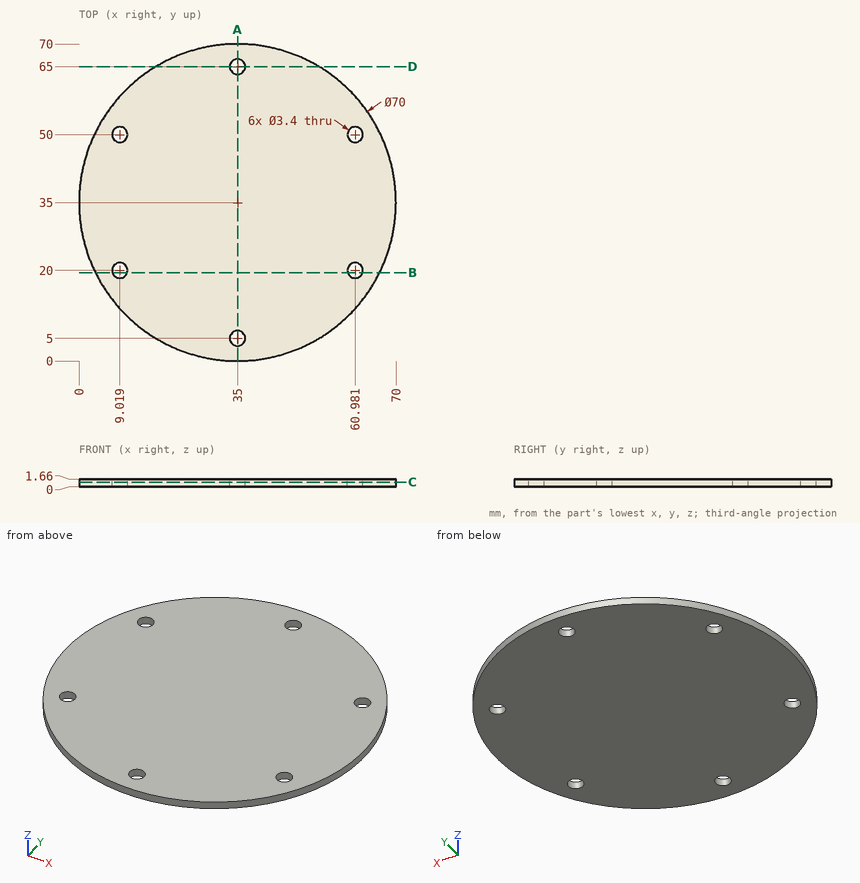
Check sheet for the drawn part. Datum: minimum x, y, z corner. Units: mm. Round coordinates to 2 decimals unless told otherwise and drop trailing zeros. Order: outer loops, then holes, each group sorted by start corner. A loop starts at its lowest first (then second) coordinate and runs counter-clockwise, first axis right, second up.
1. Section check C-C on z = 0.95. Record the cut outline in (x, y).
Final values:
outline: circle Ø70 at (35, 35); hole circle Ø3.4 at (9.02, 20); hole circle Ø3.4 at (9.02, 50); hole circle Ø3.4 at (35, 5); hole circle Ø3.4 at (35, 65); hole circle Ø3.4 at (60.98, 20); hole circle Ø3.4 at (60.98, 50)
2. Section check A-A on x = 35. Record the cut outline in (y, z).
Final values:
outline: (0, 0) - (3.3, 0) - (3.3, 1.66) - (0, 1.66) - close; (6.7, 0) - (63.3, 0) - (63.3, 1.66) - (6.7, 1.66) - close; (66.7, 0) - (70, 0) - (70, 1.66) - (66.7, 1.66) - close
3. Section check D-D on y = 65. Record the cut outline in (x, z).
Final values:
outline: (16.97, 0) - (33.3, 0) - (33.3, 1.66) - (16.97, 1.66) - close; (36.7, 0) - (53.03, 0) - (53.03, 1.66) - (36.7, 1.66) - close
4. Thickness scan on L1, parallel to X at y = 20.5, z = 0.8 (1 decimal); L2, parallel to X at y = 20, z = 0.6; L3, parallel to Y at x = 34.5, z = 0.7 (1 decimal). Record the ranges inside material, lowest first.
Final values:
L1: x = 3.1 to 7.4, 10.6 to 59.4, 62.6 to 66.9
L2: x = 3.38 to 7.32, 10.72 to 59.28, 62.68 to 66.62
L3: y = 0 to 3.4, 6.6 to 63.4, 66.6 to 70
5. Section check B-B on y = 19.5. Record the cut outline in (x, z).
Final values:
outline: (3.62, 0) - (7.39, 0) - (7.39, 1.66) - (3.62, 1.66) - close; (10.64, 0) - (59.36, 0) - (59.36, 1.66) - (10.64, 1.66) - close; (62.61, 0) - (66.38, 0) - (66.38, 1.66) - (62.61, 1.66) - close
